The listing builds one solid part. Answer for the finished solid, in the listing's coordinates (mm). Face numbers are marked on the shaded views. A direction names the side the tool comes from. Coordinates: 2 decimals unless noted, no trailing zeros. Order: outer loops, then holes, each group sorted by start corner. A loop starts at its lowest first (then second) coordinate and runs counter-clockwise, first axis right, second up. Notation, with made-up numbers: (41, 70.5) -> (58, 70.5) arc R25 cw to (58, 99.5) -> close; hole circle Ø7 at (74, 8). An arc over 180 degrees is marked (long way). Answer in a Markdown table with one row per item. Add a question column.
```python
from build123d import *

# Parameters (mm, degrees)
RESSALTO_EXTRUS_O1_DEPTH = 50
CORTE_EXTRUS_O1_DEPTH    = 50
F_3DSKETCH1_R            = 4.15
RESSALTO_EXTRUS_O2_DEPTH = 10
CHANFRO1_SIZE            = 3


with BuildPart() as part:
    # Esboço2 → Ressalto-extrusão1 (new body)
    with BuildSketch(Plane.XY):
        Polygon((0, 0), (30, 0), (30, 5), (4, 5), (4, 60), (0, 60), align=None)
    extrude(amount=RESSALTO_EXTRUS_O1_DEPTH)

    # Esboço3 → Corte-extrusão1 (cut)
    with BuildSketch(Plane(origin=(4, 0, 0), x_dir=(0, 0, -1), z_dir=(1, 0, 0))):
        with BuildLine():
            Line((-40, 37), (-10, 37))
            ThreePointArc((-10, 37), (-8, 35), (-10, 33))
            Line((-10, 33), (-40, 33))
            ThreePointArc((-40, 33), (-42, 35), (-40, 37))
        make_face()
        with BuildLine():
            Line((-40, 17), (-10, 17))
            ThreePointArc((-10, 17), (-8, 15), (-10, 13))
            Line((-10, 13), (-40, 13))
            ThreePointArc((-40, 13), (-42, 15), (-40, 17))
        make_face()
    extrude(amount=-CORTE_EXTRUS_O1_DEPTH, mode=Mode.SUBTRACT)

    # 3DSketch1 → Ressalto-extrusão2 (add)
    with BuildSketch(Plane(origin=(-9.395973154, 62.141320747, 31.218847007), x_dir=(0.493101437864631, -0.2832351206870136, -0.8225745184390569), z_dir=(0, -0.9455185755993176, 0.3255681544571544))):
        with BuildLine():
            Line((0, 0), (1.65541197, 9.862028757))
            Line((1.65541197, 9.862028757), (19.05484842, 0))
            Line((19.05484842, 0), (11.443924645, -6.486435022))
            ThreePointArc((11.443924645, -6.486435022), (3.451710065, -7.248591137), (0, 0))
        make_face()
        with Locations(Location((6.90342013, -1.158788379, 0), (0, 0, 330.45536526))):
            Circle(F_3DSKETCH1_R, mode=Mode.SUBTRACT)
    extrude(amount=RESSALTO_EXTRUS_O2_DEPTH)

    # Chanfro1
    chanfro1_edges = [part.edges().sort_by_distance(p)[0] for p in [
        (0, 60, 30.288103406),
    ]]
    chamfer(chanfro1_edges, length=CHANFRO1_SIZE)


solid = part.part
```
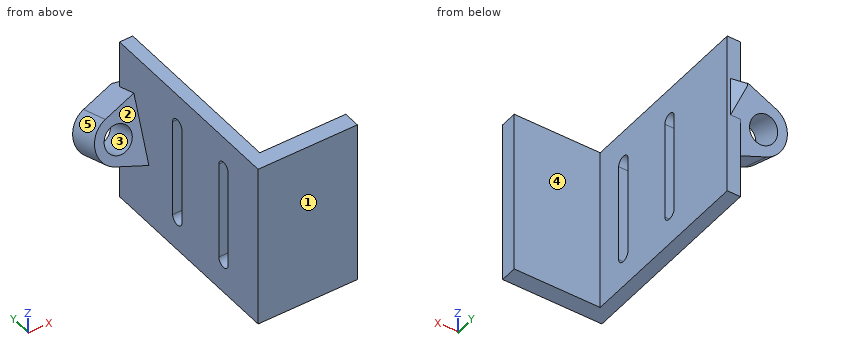
Q1. A cutting plane is placed at C-C (x = 2). Determine the outline of the cut face in (y, z), then the cut area to 3 significant figures.
Q2. Straight lines are drawn through the part: line 1 (Y direction, x = 23.5, z = 42); line 2 (Y direction, x = 3, z = 41.5); line 3 (X direction, y = 33.5, z = 46). For each, find the intervals that lie inside material, in ascending order.
Q3. A cutting plane is placed at A-A (y = 15). Determine the outline of the cut face in (x, z), then the cut area to 3 significant figures.
Q4. A cutting plane is placed at B-B (x = -8). Determine the outline of the cut face in (y, z), then the cut area to 3 significant figures.
Q5. Determine the mould class of the marked faces 1, 2 and 3 for opening direction Z: +Z half, -Z half, draft (parallel to the pull), parting line (faces both ways), or undercut.
Q6. A cutting plane is placed at D-D (z = 27). State how many separate pieces and enclosed holes the cut face has, then the cut area to 3 significant figures.
Q7. For the marked faces 4 and 5, determine the directions among +Z, -Z, +X, -X, +Y, -Y from which every point of the face is accessible in a straight line to the end or side of a thin tool.
Q8. Given pin 1 (4.5 mm diameter, centred on x = 1.5, z = 22, fed in from -Y); pin 2 (1.5 mm diameter, centred on y = 39, z = 5, fed in from +X); pin 3 (21 mm diameter, centred on x = 16, z = 36.5, fed in from +Y); pin 4 (4.5 mm diameter, centred on x = 1.5, z = 23.5, fed in from +Y), each flat-ended and moving along its own axis, determine where each tip first touches the part or whether it passes through.
Returned:
| question | item | result |
|---|---|---|
| 1 | outline | (0, 0) -> (60, 0) -> (60, 25) -> (61, 27.9) -> (61, 36) -> (60, 36.35) -> (60, 50) -> (0, 50) -> close; hole (13, 10) arc R2 ccw to (17, 10) -> (17, 40) arc R2 ccw to (13, 40) -> close; hole (33, 10) arc R2 ccw to (37, 10) -> (37, 40) arc R2 ccw to (33, 40) -> close |
| 1 | area | 2,740 mm² |
| 2 | line 1 | y = 0 to 5 |
| 2 | line 2 | y = 0 to 13.68, 16.32 to 33.68, 36.32 to 60 |
| 2 | line 3 | x = 0 to 4 |
| 3 | outline | (0, 0) -> (4, 0) -> (4, 8) -> (0, 8) -> close; (0, 42) -> (4, 42) -> (4, 50) -> (0, 50) -> close |
| 3 | area | 64.0 mm² |
| 4 | outline | (48.24, 21.56) -> (57.69, 18.3) -> (58.69, 21.19) -> (49.23, 24.45) -> close; (51.86, 32.06) -> (61.31, 28.81) -> (62.31, 31.7) -> (52.85, 34.96) -> close |
| 4 | area | 61.2 mm² |
| 5 | face 1 | draft |
| 5 | face 2 | +Z half |
| 5 | face 3 | undercut |
| 6 | separate pieces | 4 |
| 6 | enclosed holes | 0 |
| 6 | area | 402 mm² |
| 7 | face 4 | +Z, -Z, +X, +Y |
| 7 | face 5 | -X |
| 8 | pin 1 | stops at y = 0 |
| 8 | pin 2 | stops at x = 4 |
| 8 | pin 3 | stops at y = 5 |
| 8 | pin 4 | stops at y = 60.26 |
